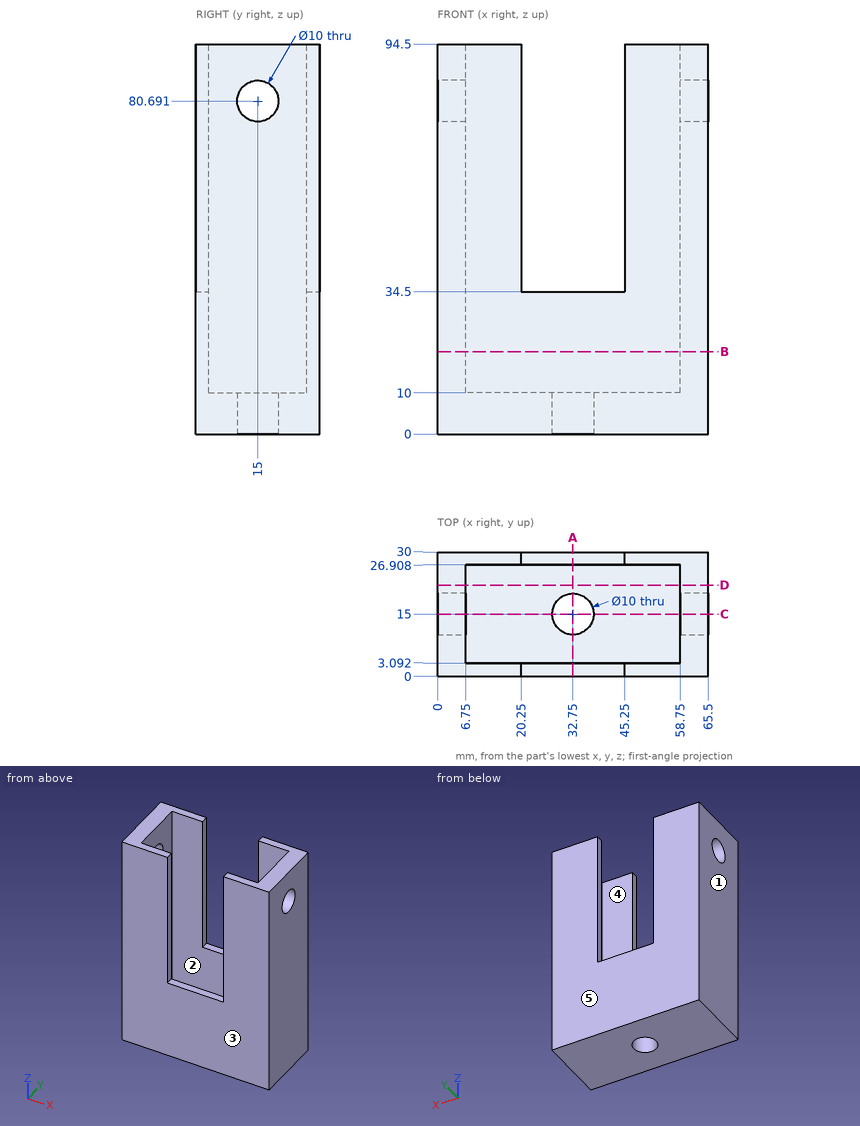
Geometry: see drawing. Coordinates: mm, zero at the bounding-box minimum. A direction names the side the tool comes from. Coordinates: 2 decimals unless noted, no trailing zeros. Loops run counter-clockwise (first coordinate to the right, second up) from the corner with the lowest first, then second, coordinate; pieces in that order, holes last.
Q1. Material intervals for line 1 (Y direction, x = 56, z = 60.5); line 2 (X direction, y = 9.75, z = 89); line 3 (Y direction, x = 32.75, z = 7.5), sorted ascending.
Q2. Draft query along Y for the marked faces 1, 2 and 3. Return one class per face: +Y half, -Y half, draft (parallel to the pull), parting line (faces both ways), or undercut.
Q3. Contact query for flat-ended pins moving along their axis: pin 1 (1.5 mm diameter, centred on x = 29.5, y = 1.5, fed in from +Z); pin 2 (12 mm diameter, centred on x = 35.5, y = 10, fed in from +Z). Output: stop coordinate, or through.
Q4. Cut plane D-D (y = 22). Output: boundary loops of the cut face in (x, z), then the cut area to 3 significant figures.
Q5. Cut plane A-A (x = 32.75). Output: boundary loops of the cut face in (y, z).
Q6. Set-up query: the marked faces 4 and 5. Return all of +Z, -Z, +X, -X, +Y, -Y with unobstructed straight access to the full face (end or side cutting, diameter ignored); none if empty.
Q7. Cut plane B-B (z = 20). Output: boundary loops of the cut face in (x, y).
Q8. Cut plane C-C (y = 15). Output: boundary loops of the cut face in (x, z), then the cut area to 3 significant figures.
Working result:
1. line 1: y = 0 to 3.09, 26.91 to 30
1. line 2: x = 0 to 6.75, 58.75 to 65.5
1. line 3: y = 0 to 10, 20 to 30
2. face 1: draft
2. face 2: undercut
2. face 3: -Y half
3. pin 1: stops at z = 34.5
3. pin 2: stops at z = 10
4. outline: (0, 0) - (65.5, 0) - (65.5, 94.5) - (58.75, 94.5) - (58.75, 10) - (6.75, 10) - (6.75, 94.5) - (0, 94.5) - close
4. area: 1,800 mm2
5. outline: (0, 0) - (10, 0) - (10, 10) - (3.09, 10) - (3.09, 34.5) - (0, 34.5) - close; (20, 0) - (30, 0) - (30, 34.5) - (26.91, 34.5) - (26.91, 10) - (20, 10) - close
6. face 4: +Z
6. face 5: +Z, -Z, +X, -X, +Y
7. outline: (0, 0) - (65.5, 0) - (65.5, 30) - (0, 30) - close; hole (6.75, 3.09) - (58.75, 3.09) - (58.75, 26.91) - (6.75, 26.91) - close
8. outline: (0, 0) - (27.75, 0) - (27.75, 10) - (6.75, 10) - (6.75, 75.69) - (0, 75.69) - close; (0, 85.69) - (6.75, 85.69) - (6.75, 94.5) - (0, 94.5) - close; (37.75, 0) - (65.5, 0) - (65.5, 75.69) - (58.75, 75.69) - (58.75, 10) - (37.75, 10) - close; (58.75, 85.69) - (65.5, 85.69) - (65.5, 94.5) - (58.75, 94.5) - close
8. area: 1,560 mm2
